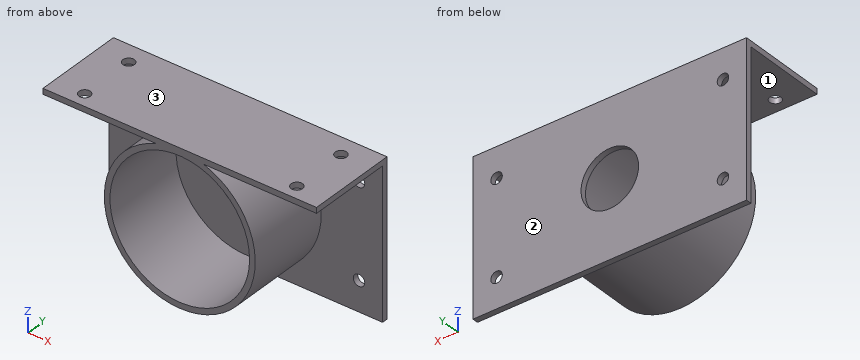
Autodesk Inventor part; units mm, degrees
ref_plane "YZ Plane" through (0, 0, 0) normal (1, 0, 0) x (0, 1, 0)
ref_plane "XZ Plane" through (0, 0, 0) normal (0, 1, 0) x (-1, 0, 0)
ref_plane "XY Plane" through (0, 0, 0) normal (0, 0, 1) x (1, 0, 0)
sketch "Sketch1" plane through (0, 0, 0) normal (0, 1, 0) x (-1, 0, 0)
  circle A0 centre (0, 0) radius 15.25
  circle A1 centre (0, 0) radius 32.5 construction
  line L0 (0, 0) -> (0, -32.5) construction
  line L1 (0, 0) -> (-22.981, -22.981) construction
  circle A2 centre (-22.981, -22.981) radius 3.05 construction
  circle A3 centre (22.981, -22.981) radius 3.05 construction
  circle A4 centre (22.981, 22.981) radius 3.05 construction
  circle A5 centre (-22.981, 22.981) radius 3.05 construction
  circle A6 centre (0, 0) radius 40
  circle A7 centre (22.981, -22.981) radius 5 construction
  dimension "d0" = 30.5
  dimension "d1" = 6.1
  dimension "d3" = 45
  dimension "d4" = 65
  dimension "d7" = 360
  dimension "d9" = 80
  dimension "d10" = 10
extrude "Extrusion1" add sketch "Sketch1" along normal blind 3
sketch "Sketch2" plane through (0, 0, 0) normal (0, -1, 0) x (1, 0, 0)
  circle A0 centre (0, 0) radius 40
  circle A1 centre (0, 0) radius 37
  dimension "d13" = 3
extrude "Extrusion2" add sketch "Sketch2" along normal blind 45
sketch "Sketch3" plane through (0, 3, 0) normal (0, 1, 0) x (1, 0, 0)
  line L0 (-72.5, -41) -> (72.5, -41)
  line L1 (72.5, -41) -> (72.5, 41)
  line L2 (72.5, 41) -> (-72.5, 41)
  line L3 (-72.5, 41) -> (-72.5, -41)
  line L4 (-72.5, -41) -> (72.5, 41) construction
  line L5 (72.5, -41) -> (-72.5, 41) construction
  circle A0 centre (0, 0) radius 40
  circle A1 centre (0, 0) radius 15.25
  line L6 (-60, -25) -> (60, -25) construction
  line L7 (60, -25) -> (60, 25) construction
  line L8 (60, 25) -> (-60, 25) construction
  line L9 (-60, 25) -> (-60, -25) construction
  line L10 (-60, -25) -> (60, 25) construction
  line L11 (60, -25) -> (-60, 25) construction
  circle A2 centre (-60, 25) radius 3.05
  circle A3 centre (-60, -25) radius 3.05
  circle A4 centre (60, 25) radius 3.05
  circle A5 centre (60, -25) radius 3.05
  dimension "d16" = 145
  dimension "d17" = 82
  dimension "d18" = 120
  dimension "d19" = 50
  dimension "d20" = 6.1
extrude "Extrusion3" add sketch "Sketch3" against normal blind 3 contours L3 L2 L1 L0
sketch "Sketch4" plane through (-72.5, 3, 41) normal (0, 0, 1) x (1, 0, 0)
  line L0 (32.5, -3) -> (112.5, -3)
  line L1 (32.5, -48) -> (112.5, -48)
  line L2 (0, 0) -> (145, 0)
  line L3 (0, 0) -> (0, -3)
  line L4 (145, -3) -> (0, -3)
  line L5 (145, 0) -> (145, -3)
  line L6 (0, 0) -> (0, -3)
  line L7 (32.5, -48) -> (112.5, -48)
  line L8 (0, -3) -> (32.5, -3)
  line L9 (32.5, -3) -> (32.5, -48)
  line L10 (32.5, -48) -> (0, -48)
  line L11 (0, -48) -> (0, -3)
  line L12 (112.5, -48) -> (145, -48)
  line L13 (145, -48) -> (145, -3)
  line L14 (145, -3) -> (112.5, -3)
  line L15 (112.5, -3) -> (112.5, -48)
  line L16 (16.25, -48) -> (16.25, -3) construction
  line L17 (145, -3) -> (0, -3)
  line L18 (128.75, -48) -> (128.75, -3) construction
  circle A0 centre (16.25, -40.5) radius 3.05
  line L19 (16.25, -40.5) -> (128.75, -40.5) construction
  line L20 (128.75, -40.5) -> (128.75, -10.5) construction
  line L21 (128.75, -10.5) -> (16.25, -10.5) construction
  line L22 (16.25, -10.5) -> (16.25, -40.5) construction
  circle A1 centre (16.25, -10.5) radius 3.05
  circle A2 centre (128.75, -10.5) radius 3.05
  circle A3 centre (128.75, -40.5) radius 3.05
  point P0 (72.5, -3)
  dimension "d23" = 30
  dimension "d24" = 7.5
  dimension "d25" = 6.1
extrude "Extrusion4" add sketch "Sketch4" against normal blind 3 contours L9 L10 L11 L4 | L0 L15 L1 L9 | L4 L13 L12 L15
properties part number "WheelHolder" material "Aluminum 6061-AHC"
Geometry check sheet. Reference: the model listing, model coordinates, mm. Face numbers are marked on the shaded views. Round coordinates to 2 decimals unless told otherwise and drop trailing zeros. Write each loop counter-clockwise with the first axis right and the second up, starting at its lowest first coordinate (ties: lowest second). Pieces come first, ordered by that corner, then holes.
Item 1: Mould release check, pull along Z, two halves, no side actions. Record for the marked faces 1, 2 and 3: +Z half, -Z half, draft (parallel to the pull), parting line (faces both ways), or undercut.
Determined:
face 1: undercut
face 2: draft
face 3: +Z half
Item 2: Go/stop test with flat-tipped pins: pin 1 Ø1.5 at (y, z) = (-2.5, -30.5) entering from +X; pin 2 Ø22 at (x, z) = (15, -5) entering from -Y; pin 3 Ø8 at (x, y) = (56.25, -37.5) entering from -Z; pin 4 Ø5.5 at (x, z) = (-60, 25) entering from +Y. Record where each tip stops, or that it passes through.
Determined:
pin 1: stops at x = 26.74
pin 2: stops at y = 0
pin 3: stops at z = 38
pin 4: passes through
Item 3: Section check D-D (y = -31.5). Record the boundary of the cut face in (x, z), plus the area to 3 significant figures.
Determined:
outline: (-72.5, 38) - (-12.49, 38) arc R40 ccw (long way) to (12.49, 38) - (72.5, 38) - (72.5, 41) - (-72.5, 41) - close; hole circle Ø74 at (0, 0)
area: 1,130 mm2
Item 4: Section check B-B (z = 0). Record the boundary of the cut face in (x, y).
Determined:
outline: (-72.5, 0) - (-40, 0) - (-40, -45) - (-37, -45) - (-37, 0) - (-15.25, 0) - (-15.25, 3) - (-72.5, 3) - close; (15.25, 0) - (37, 0) - (37, -45) - (40, -45) - (40, 0) - (72.5, 0) - (72.5, 3) - (15.25, 3) - close
Item 5: Section check A-A (y = -7.5). Record the boundary of the cut face in (x, z), plus the area to 3 significant figures.
Determined:
outline: (-72.5, 38) - (-59.3, 38) - (-59.3, 41) - (-72.5, 41) - close; (-53.2, 38) - (-12.49, 38) arc R40 ccw (long way) to (12.49, 38) - (53.2, 38) - (53.2, 41) - (-53.2, 41) - close; (59.3, 38) - (72.5, 38) - (72.5, 41) - (59.3, 41) - close; hole circle Ø74 at (0, 0)
area: 1,090 mm2
Item 6: Material ranges on line 1 along Z through (x, y) = (-60, 2.4); line 2 along X through (y, z) = (1.55, 25); line 3 along Z through (x, y) = (-20.5, -6), recorded low to high.
Determined:
line 1: z = -41 to -28.05, -21.95 to 21.95, 28.05 to 41
line 2: x = -72.5 to -63.05, -56.95 to 56.95, 63.05 to 72.5
line 3: z = -34.35 to -30.8, 30.8 to 34.35, 38 to 41
Item 7: Section check C-C (x = 0). Record the boundary of the cut face in (y, z), plus the area to 4 significant figures.
Determined:
outline: (-45, -40) - (0, -40) - (0, -41) - (3, -41) - (3, -15.25) - (0, -15.25) - (0, -37) - (-45, -37) - close; (-45, 37) - (0, 37) - (0, 15.25) - (3, 15.25) - (3, 41) - (-45, 41) - close
area: 469.5 mm2
